Design review of the part built by this model. Coordinates are the model's own, in mm. Face numbers are marked on the shaded views. Give positions to 0.01 mm unless a question says otherwise; leave off trailing zeros. Write each loop counter-clockwise with the first axis right and the second up, starting at its lowest first coordinate (ties: lowest second). Pieces come first, ordered by that corner, then holes. Notation, with made-up numbers: (19, 7) -> (26, 7) arc R24 cw to (26, 32) -> close; hole circle Ø8 at (-12, 77). An arc over 180 degrees is marked (long way). Answer as a JSON object with one key per item and string values.
```python
from build123d import *

# Parameters (mm, degrees)
F0_R     = 6.35
F1_DEPTH = 50
F2_R     = 1.5875
F3_DEPTH = 12.5
F4_R     = 4.7625
F5_DEPTH = 25


with BuildPart() as f1:
    # F0 (on Front) → F1 (new body)
    with BuildSketch(Plane.XZ):
        Circle(F0_R)
    extrude(amount=F1_DEPTH)

    # F2 (on Right) → F3 (cut, symmetric)
    with BuildSketch(Plane.YZ):
        with Locations((-10, 0)):
            Circle(F2_R)
        with Locations((-40, 0)):
            Circle(F2_R)
    extrude(amount=F3_DEPTH, both=True, mode=Mode.SUBTRACT)

    # F4 (on face) → F5 (cut)
    with BuildSketch(Plane.XZ.offset(50)):
        Circle(F4_R)
    extrude(amount=-F5_DEPTH, mode=Mode.SUBTRACT)


solid = f1.part
```
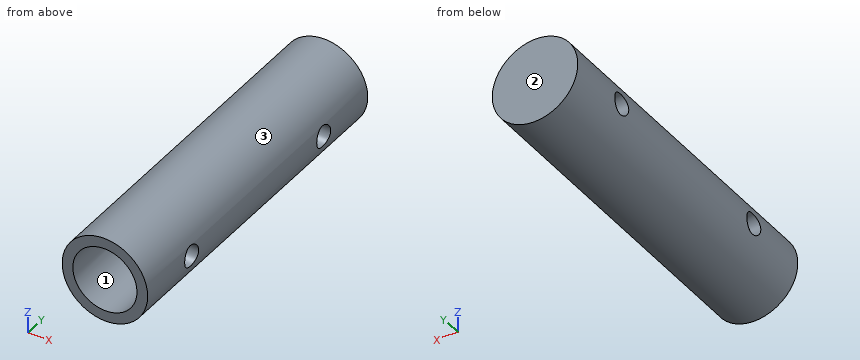
(1) We need section B-B, the plane x = 2. State the section outline as (y, z) points (1 decimal), then the cut area to 3 significant figures.
Here are the results:
{"outline": "(-50, -6) -> (0, -6) -> (0, 6) -> (-50, 6) -> (-50, 4.3) -> (-25, 4.3) -> (-25, -4.3) -> (-50, -4.3) -> close; hole circle Ø3.2 at (-10, 0)", "area": "379 mm²"}
(2) For line 1 along Y through (x, z) = (5.4, 0); line 2 along Z through (x, y) = (0, -34), list the stretches that pass through material, from the lowest coordinate up.
Here are the results:
{"line 1": "y = -50 to -41.59, -38.41 to -11.59, -8.41 to 0", "line 2": "z = -6.35 to -4.76, 4.76 to 6.35"}
(3) The part is to be moulded in two halves that separate along X. For the marked faces 1, 2 and 3, say which applies: +X half, -X half, draft (parallel to the pull), parting line (faces both ways), or undercut.
Here are the results:
{"face 1": "undercut", "face 2": "draft", "face 3": "parting line"}
(4) We need section C-C, the plane z = -0.5. State the section outline as (x, y) points.
Here are the results:
{"outline": "(-6.33, -50) -> (-4.74, -50) -> (-4.74, -41.51) -> (-6.33, -41.51) -> close; (-6.33, -38.49) -> (-4.74, -38.49) -> (-4.74, -25) -> (4.74, -25) -> (4.74, -38.49) -> (6.33, -38.49) -> (6.33, -11.51) -> (-6.33, -11.51) -> close; (-6.33, -8.49) -> (6.33, -8.49) -> (6.33, 0) -> (-6.33, 0) -> close; (4.74, -50) -> (6.33, -50) -> (6.33, -41.51) -> (4.74, -41.51) -> close"}
(5) We need section D-D, the plane z = 4. State the section outline as (x, y) points.
Here are the results:
{"outline": "(-4.93, -50) -> (-2.58, -50) -> (-2.58, -25) -> (2.58, -25) -> (2.58, -50) -> (4.93, -50) -> (4.93, 0) -> (-4.93, 0) -> close"}
(6) Clearance check with flat-ended pins moving along their axes: pin 1 (1.5 mm diameter, centred on y = -42.5, z = 4, fed in from -X); pin 2 (4 mm diameter, centred on x = 2.5, y = -13, fed in from -Z); pin 3 (6 mm diameter, centred on x = -5, y = -7.5, fed in from -Z). State where each tip first meets the part, or that it passes through.
Here are the results:
{"pin 1": "stops at x = -5.46", "pin 2": "stops at z = -6.33", "pin 3": "stops at z = -6.03"}
